from build123d import *

# Parameters (mm, degrees)
SWEEP_THIN1_PROFILE_R   = 5.97
SWEEP_THIN1_PROFILE_R_2 = 5.57
FILLET1_R               = 1


with BuildPart() as part:
    # Sweep-Thin1: sweep along a path in Sketch1
    with BuildLine(Plane(origin=(0, 0, 0), x_dir=(0, 1, 0), z_dir=(0, 0, 1))) as sweep_thin1_path:
        Line((13.335, 0), (150, 0))
        ThreePointArc((150, 0), (185, 35), (150, 70))
        Line((150, 70), (-184.185, 70))
    # Sweep-Thin1 profile (on start of the path) → Sweep-Thin1 (sweep)
    with BuildSketch(Plane.ZX.offset(13.335)):
        Circle(SWEEP_THIN1_PROFILE_R)
        Circle(SWEEP_THIN1_PROFILE_R_2, mode=Mode.SUBTRACT)
    sweep(path=sweep_thin1_path.line)

    # Sketch19 → Revolve2 (revolve)
    with BuildSketch(Plane(origin=(0, 0, 0), x_dir=(0, 1, 0), z_dir=(0, 0, 1)), mode=Mode.PRIVATE) as revolve2_sk:
        Polygon((-184.185, 76.37), (-218.06, 76.37), (-218.06, 74.891814615), (-186.185, 74.023934498), (-186.185, 72.908200054), (-184.185, 75.57), align=None)
    revolve(revolve2_sk.sketch.rotate(Axis((-70, -184.185, 0), (0, -1, 0)), 270), axis=Axis((-70, -184.185, 0), (0, -1, 0)))

    # Fillet1
    # the kernel refuses this fillet: 1 mm, written as the material it takes off along each edge
    with BuildSketch(Plane(origin=(-70, -184.185, 0), x_dir=(0, 0, 1), z_dir=(1, 0, 0))) as fillet1_piece_1:
        with BuildLine():
            CenterArc((5.37, 0.8), FILLET1_R, 306.869897646, 53.130102354)
            Line((6.37, 0.8), (6.39, 0.8))
            Line((6.39, 0.8), (6.39, 0))
            Line((6.39, 0), (6.37, -0.02))
            ThreePointArc((6.37, -0.02), (6.17, -0.02), (5.982, -0.016))
            Line((5.982, -0.016), (5.97, 0))
        make_face()
    revolve(axis=Axis((-70, -184.185, 0), (0, -1, 0)), mode=Mode.SUBTRACT)


solid = part.part
Part model, mm, in its own coordinate system. A direction names the side the tool comes from. Coordinates: 2 decimals unless noted, no trailing zeros. Write each loop counter-clockwise with the first axis right and the second up, starting at its lowest first coordinate (ties: lowest second). Pieces come first, ordered by that corner, then holes. Notation, with made-up numbers: (43, 24.25) - (92, 24.25) arc R27 ccw to (92, 46.25) - close; hole circle Ø4 at (89.5, 32). An arc over 180 degrees is marked (long way). Put each result on its own line as item: value.
1. 3-axis set-ups, long thin cutter, end or side, ignore diameter. For faces 4 (the cylindrical face through (-64.562, -19.432, -1.207)), 5 (the conical face through (-65.654, -201.899, -0.965)): which of +Z, -Z, +X, -X, +Y, -Y reach the whole face in a straight line?
Final values:
face 4: none
face 5: -Y
2. Probe line 1 along X through (y, z) = (82, 0); line 2 along X through (y, z) = (-80.5, 0); line 3 along Z through (x, y) = (-70, -73.5). List the from-to ranges inside material, lowest first. Write a range as [from, to].
Final values:
line 1: x = [-75.97, -75.57], [-64.43, -64.03], [-5.97, -5.57], [5.57, 5.97]
line 2: x = [-75.97, -75.57], [-64.43, -64.03]
line 3: z = [-5.97, -5.57], [5.57, 5.97]
3. Band-saw the part on D-D (x = -35). Write the cut outline in (y, z), then the cut area to 3 significant figures.
Final values:
outline: circle Ø11.94 at (185, 0); hole circle Ø11.14 at (185, 0)
area: 14.5 mm²
4. Two-plate mould, pull along Z, no slides. Class faces 1 (the cylindrical face through (-5.438, 82.624, -1.207)), 2 (the cylindrical face through (-5.83, 82.62, -1.29)), 3 (the flat face through (-65, -218.06, -1)): +Z half, -Z half, draft (parallel to the pull), parting line (faces both ways), or undercut.
Final values:
face 1: undercut
face 2: parting line
face 3: draft
5. Band-saw the part on C-C (y = -163). Write the cut outline in (x, z), then the cut area to 3 significant figures.
Final values:
outline: circle Ø11.94 at (-70, 0); hole circle Ø11.14 at (-70, 0)
area: 14.5 mm²
6. Band-saw the part on A-A (y = 56). Write the cut outline in (x, z), then the cut area to 3 significant figures.
Final values:
outline: circle Ø11.94 at (-70, 0); circle Ø11.94 at (0, 0); hole circle Ø11.14 at (-70, 0); hole circle Ø11.14 at (0, 0)
area: 29.0 mm²
7. Flat gauge pins, fed straight in: pin 1 Ø6 at (x, z) = (-23.5, 1) entering from -Y; pin 2 Ø1 at (y, z) = (-25.5, -2) entering from +X; pin 3 Ø4 at (y, z) = (-45.5, -5) entering from +X. Where does each tip first touch, or does it go through?
Final values:
pin 1: stops at y = 175.2
pin 2: stops at x = -64.22
pin 3: stops at x = -64.84
8. Band-saw the part on B-B (z = 0). Write the cut outline in (x, y) (3 decimals).
Final values:
outline: (-76.37, -218.06) - (-74.892, -218.06) - (-74.024, -186.185) - (-72.908, -186.185) - (-75.57, -184.185) - (-75.57, 150) arc R40.57 cw to (5.57, 150) - (5.57, 13.335) - (5.97, 13.335) - (5.97, 150) arc R40.97 ccw to (-75.97, 150) - (-75.97, -184.185) arc R1 ccw to (-76.37, -184.985) - close; (-67.092, -186.185) - (-65.976, -186.185) - (-65.108, -218.06) - (-63.63, -218.06) - (-63.63, -184.985) arc R1 ccw to (-64.03, -184.185) - (-64.03, 150) arc R29.03 cw to (-5.97, 150) - (-5.97, 13.335) - (-5.57, 13.335) - (-5.57, 150) arc R29.43 ccw to (-64.43, 150) - (-64.43, -184.185) - close
